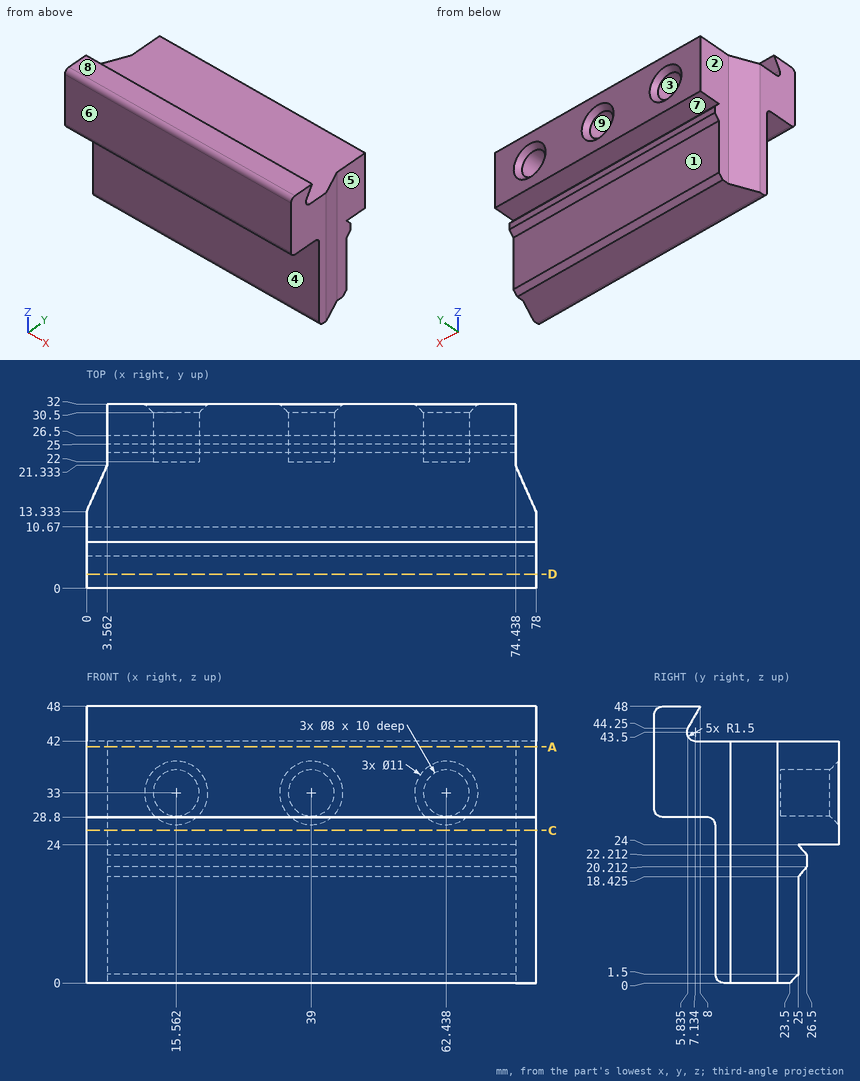
Study the drawing (mm; zero at the part's minimum x, y, z) and answer. A direction names the side the tool comes from. Give positions to 0.01 mm unless a question says otherwise; leave off trailing zeros. Write each loop counter-clockwise with the first axis right and the second up, starting at its lowest first coordinate (ties: lowest second). Pieces come first, ordered by that corner, then holes. Notation, with made-up numbers: M 45.5,19.25 L 65.5,19.25 A6 cw 65.5,24.25 Z; hole C 23.25,62.5 d4. An arc over 180 degrees is marked long. Put each result on its own line as item: value. Start each with the question number.
1. Consider line 1 along X through (y, z) = (28, 33); line 2 along Z through (x, y) = (39, 27.5); line 3 along Z through (x, y) = (10, 12). Determine where each line is inside the solid, lowest interval first.
2. Which of the six approach directions +Z, -Z, +X, -X, +Y, -Y give full straight-line access (tool end or side, diameter ignored) to the marked faces 1, 2, 3, 4 and 5?
3. The part is cut by section D-D, the plane y = 2.5. Give the vertices of the cut face in (x, z), and give its area (3 significant figures).
4. The part is cut by section A-A, the plane z = 41. Give the vertices of the cut face in (x, y).
5. Each of these flat-tipped pins is pushed along its axis until it touches: pin 1 Ø4 at (x, y) = (11, 25.5) entering from +Z; pin 2 Ø2.5 at (x, z) = (62.5, 34.5) entering from +Y; pin 3 Ø6 at (x, y) = (38.5, 6) entering from -Z. Where does it stop, or does it pass through?
6. For a pull along Z with two mould halves and no side action, classify the marked faces 6, 7, 8 and 9 as released by +Z, released by -Z, zero draft, split by the parting line, or undercut.
7. The part is cut by section C-C, the plane z = 26.5. Give the vertices of the cut face in (x, y), and give its area (3 significant figures).
Final values:
1. line 1: x = 3.56 to 11.56, 19.56 to 35, 43 to 58.44, 66.44 to 74.44
1. line 2: z = 24 to 29, 37 to 42
1. line 3: z = 0.01 to 42
2. face 1: -Z, +X, -X, +Y
2. face 2: +Z, -Z, -X, +Y
2. face 3: +Y
2. face 4: -Z, +X, -X, -Y
2. face 5: +Z, -Z, +X, +Y
3. outline: M 0,28.8 L 78,28.8 L 78,48 L 0,48 Z
3. area: 1,500 mm²
4. outline: M 0,0 L 78,0 L 78,13.33 L 74.44,21.33 L 74.44,32 L 3.56,32 L 3.56,21.33 L 0,13.33 Z
5. pin 1: stops at z = 42
5. pin 2: stops at y = 22
5. pin 3: stops at z = 28.8
6. face 6: zero draft
6. face 7: undercut
6. face 8: released by +Z
6. face 9: undercut
7. outline: M 0,10.67 L 78,10.67 L 78,13.33 L 74.44,21.33 L 74.44,32 L 3.56,32 L 3.56,21.33 L 0,13.33 Z
7. area: 1,560 mm²
